Source: CAD feature listing. Evaluate the final solid. Frame: model axes, mm. A direction names the side the tool comes from. Give positions to 0.01 mm unless a question says otherwise; leave off trailing zeros. Loops run counter-clockwise (first coordinate to the right, second up) from the corner with the lowest first, then second, coordinate; pieces in that order, holes last. Notation, with made-up numbers: (69.25, -9.75) -> (79.25, -9.75) arc R11 cw to (79.25, 3.25) -> close; hole circle Ø2 at (68, -26). An arc over 180 degrees is marked (long way). Return JSON: item names as keys, results as strings. Group by question number.
(1) Cut plane A-A on z = 2.5. Give the number of separate pieces and of enclosed holes in the cut face, then the cut area to 3 significant figures.
(2) Ray query, line 1 (Y direction, x = 0, z = 1.3) (3 decimals); line 2 (Y direction, x = 1, z = 1.75); line 3 (Z direction, x = -6, y = 13.5) (3 decimals). Return the intervals inside material, ascending. Write a range as from..to.
(3) Cut plane C-C on x = -26.67. Return loops of the section in (y, z) (3 decimals), then the cut area to 3 significant figures.
(4) Cut plane D-D on y = -12.5. Return loops of the section in (x, z) (3 decimals), then the cut area to 3 significant figures.
(5) Access query for faces 5 (the face through (-26.74, 3.174, 14.132)), 6 (the face through (-20.43, -11.6, 14.13)), 7 (the face through (-6.35, 19, 2)). Directions: +Z, -Z, +X, -X, +Y, -Y. A direction counts if a zero-diameter tool reaches every point of the face in a straight line with its end or side. Return the directions, or none.
(6) Pin query (flat end, axial travel): pin 1 (4 mm diameter, centred on y = -2.5, z = 7, fed in from -X); pin 2 (10 mm diameter, centred on x = -8, y = -21.5, fed in from +Z); pin 3 (1 mm diameter, centred on x = -23, z = 1, fed in from +Y); pin 4 (1 mm diameter, centred on y = 15, z = 1.5, fed in from -X). Return the tip coordinate at first contact, or that it passes through.
(7) Draft query along Y for faces 1 (the face through (0, 31.75, 2)), 2 (the face through (-0.41, 28.55, 1.61)), 3 (the face through (-25.736, -15.112, 14.132)), 4 (the face through (6.35, 0, 2)). Return one class per face: released by +Y, released by -Y, zero draft, split by the parting line, or undercut.
(8) Cut plane B-B on y = 25.4. Return loops of the section in (x, z) (3 decimals), then the cut area to 3 significant figures.
```python
from build123d import *

# Parameters (mm, degrees)
BOSS_EXTRUDE1_DEPTH = 3.175
SKETCH4_R           = 3.96875
SKETCH4_R_2         = 3.175
CUT_EXTRUDE1_DEPTH  = 4.175
BOSS_EXTRUDE3_DEPTH = 22.225


with BuildPart() as part:
    # Sketch1 → Boss-Extrude1 (new body)
    with BuildSketch(Plane.XY):
        with BuildLine():
            Line((-31.75, 0), (-31.75, 6.35))
            Line((-31.75, 6.35), (-6.35, 6.35))
            Line((-6.35, 6.35), (-6.35, 31.75))
            Line((-6.35, 31.75), (6.35, 31.75))
            Line((6.35, 31.75), (6.35, 6.35))
            Line((6.35, 6.35), (6.35, -31.75))
            Line((6.35, -31.75), (0, -31.75))
            ThreePointArc((0, -31.75), (-22.450640303, -22.450640303), (-31.75, 0))
        make_face()
    extrude(amount=BOSS_EXTRUDE1_DEPTH)

    # Sketch4 → Cut-Extrude1 (cut, through all)
    with BuildSketch(Plane.XY.offset(3.175)):
        Circle(SKETCH4_R)
        with Locations((0, 25.4)):
            Circle(SKETCH4_R_2)
    extrude(amount=-CUT_EXTRUDE1_DEPTH, mode=Mode.SUBTRACT)

    # Sketch6 → Boss-Extrude3 (add)
    with BuildSketch(Plane.XY.offset(3.175)):
        with BuildLine():
            ThreePointArc((-29.845, 0), (-26.67, 3.175), (-23.495, 0))
            ThreePointArc((-23.495, 0), (-20.347266862, -11.7475), (-11.7475, -20.347266862))
            ThreePointArc((-11.7475, -20.347266862), (-10.585369343, -24.684397519), (-14.9225, -25.846528176))
            ThreePointArc((-14.9225, -25.846528176), (-25.846528176, -14.9225), (-29.845, 0))
        make_face()
    extrude(amount=BOSS_EXTRUDE3_DEPTH)


solid = part.part
```
Answers:
{
 "1": {"separate pieces": "1", "enclosed holes": "2", "area": "1,480 mm²"},
 "2": {"line 1": "-31.75..-3.969, 3.969..22.225, 28.575..31.75", "line 2": "-31.75..-3.84, 3.84..22.39, 28.41..31.75", "line 3": "0..3.175"},
 "3": {"outline": "(-17.227, 0) -> (6.35, 0) -> (6.35, 3.175) -> (3.175, 3.175) -> (3.175, 25.4) -> (-13.395, 25.4) -> (-13.395, 3.175) -> (-17.227, 3.175) -> close", "area": "443 mm²"},
 "4": {"outline": "(-29.186, 0) -> (6.35, 0) -> (6.35, 3.175) -> (-19.894, 3.175) -> (-19.894, 25.4) -> (-27.101, 25.4) -> (-27.101, 3.175) -> (-29.186, 3.175) -> close", "area": "273 mm²"},
 "5": {"face 5": "+Z, +Y", "face 6": "+Z, +X, +Y", "face 7": "+Z, -Z, -X, +Y"},
 "6": {"pin 1": "x = -29.84", "pin 2": "z = 25.4", "pin 3": "y = 6.35", "pin 4": "x = -6.35"},
 "7": {"face 1": "released by +Y", "face 2": "undercut", "face 3": "released by -Y", "face 4": "zero draft"},
 "8": {"outline": "(-6.35, 0) -> (-3.175, 0) -> (-3.175, 3.175) -> (-6.35, 3.175) -> close; (3.175, 0) -> (6.35, 0) -> (6.35, 3.175) -> (3.175, 3.175) -> close", "area": "20.2 mm²"}
}
